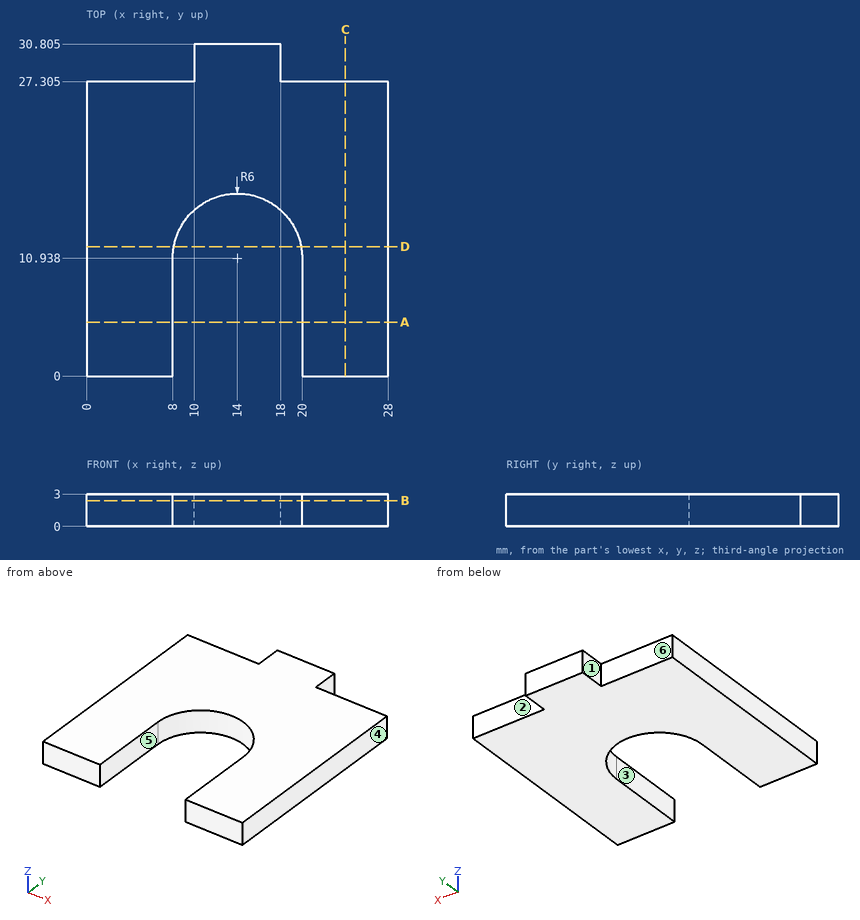
Job drawing, mm, ordinate dimensions from the low corner. One solid piece. A direction names the side the tool comes from. Give positions to 0.01 mm unless a question says otherwise; leave off trailing zeros. Loops run counter-clockwise (first coordinate to the right, second up) from the corner with the lowest first, then second, coordinate; pieces in that order, holes last. Notation, with made-up numbers: M 47.5,86.25 L 69.5,86.25 A15 ccw 69.5,91.25 Z; hole C 19,-20 d6. An arc over 180 degrees is marked long. Use one line per item in the form item = value.
Item 1: Slice it at B-B on z = 2.4. List the corners of the cut face in (x, y) (1 decimal), and give its area (3 significant figures).
Filled in:
outline = M 0,0 L 8,0 L 8,10.9 A6 cw 20,10.9 L 20,0 L 28,0 L 28,27.3 L 18,27.3 L 18,30.8 L 10,30.8 L 10,27.3 L 0,27.3 Z
area = 605 mm^2
Item 2: Which spindle directions (+Z, -Z, +X, -X, +Y, -Y) get a long thin tool onto all of the face, cutting with end or side? Do the marked faces 4, 5 and 6. Say none if no direction does.
Filled in:
face_4 = +Z, -Z, +X, +Y, -Y
face_5 = +Z, -Z, -Y
face_6 = +Z, -Z, -X, +Y
Item 3: Drill centre lines: L1, parallel to X at y = 7.5, z = 2.6; L2, parallel to X at y = 29, z = 1.35; L3, parallel to Y at x = 4.5, z = 2.75 (1 decimal). Where is each one in solid material? Low to high.
Filled in:
L1 = 0 to 8, 20 to 28
L2 = 10 to 18
L3 = 0 to 27.3
Item 4: Slice it at D-D on y = 12. List the corners of the cut face in (x, z) (1 decimal).
Filled in:
outline = M 0,0 L 8.1,0 L 8.1,3 L 0,3 Z; M 19.9,0 L 28,0 L 28,3 L 19.9,3 Z
Item 5: Two-plate mould, pull along X, no slides. Class the marked faces 1, 2 and 3: released by +X, released by -X, zero draft, split by the parting line, or undercut.
Filled in:
face_1 = released by -X
face_2 = zero draft
face_3 = undercut
Item 6: Flat gauge pins, fed straight in: pin 1 Ø1.5 at (y, z) = (29.5, 1.5) entering from -X; pin 2 Ø1 at (x, z) = (21.5, 2) entering from +Y (1 decimal). Where does each tip first touch, or does it go through?
Filled in:
pin_1 = 10
pin_2 = 27.3
Item 7: Slice it at C-C on x = 24. List the corners of the cut face in (y, z) (1 decimal).
Filled in:
outline = M 0,0 L 27.3,0 L 27.3,3 L 0,3 Z
Item 8: Slice it at A-A on y = 5. List the corners of the cut face in (x, z), and give its area (3 significant figures).
Filled in:
outline = M 0,0 L 8,0 L 8,3 L 0,3 Z; M 20,0 L 28,0 L 28,3 L 20,3 Z
area = 48.0 mm^2
